```python
from build123d import *

# Parameters (mm, degrees)
SCHIZZO1_R                   = 10
ESTRUSIONE_ESTRUSIONE1_DEPTH = 20
SCHIZZO2_R                   = 3
ESTRUSIONE_ESTRUSIONE2_DEPTH = 13.2
SMUSSO1_SIZE                 = 0.5
FORO_FILETTATO_M10_3_D       = 8.5


with BuildPart() as part:
    # Schizzo1 → Estrusione-Estrusione1 (new body)
    with BuildSketch(Plane.XY):
        Circle(SCHIZZO1_R)
    extrude(amount=ESTRUSIONE_ESTRUSIONE1_DEPTH)

    # Schizzo2 → Estrusione-Estrusione2 (add, symmetric)
    with BuildSketch(Plane.XY.offset(10)):
        Circle(SCHIZZO2_R)
    extrude(amount=ESTRUSIONE_ESTRUSIONE2_DEPTH, both=True)

    # Smusso1
    smusso1_edges = [part.edges().sort_by_distance(p)[0] for p in [
        (-3, 0, -3.2),
        (-3, 0, 23.2),
    ]]
    chamfer(smusso1_edges, length=SMUSSO1_SIZE)

    # Foro filettato M10-3 (through all)
    with Locations(Plane(origin=(0, 10, 10), x_dir=(1, 0, 0), z_dir=(0, 1, 0))):
        with Locations((0, 0)):
            Hole(FORO_FILETTATO_M10_3_D / 2)


solid = part.part
```
Could you check a few things on this model? Use its own coordinates, in mm. A direction names the side the tool comes from. Round coordinates to 2 decimals unless told otherwise and drop trailing zeros. Loops run counter-clockwise (first coordinate to the right, second up) from the corner with the lowest first, then second, coordinate; pieces in that order, holes last. Notation, with made-up numbers: (45.5, -37) - (91.5, -37) arc R6 cw to (91.5, -31) - close; hole circle Ø5 at (32.5, -32). An arc over 180 degrees is marked (long way). Answer in a Markdown table with one row per item. Add a question column.
(1) If we section it at D-D (y = -6): Please give me the cut outline in (x, z), plus the area to 3 significant figures.
(2) I'm going to push flat-ended pins straight in: pin 1 (8 mm diameter, centred on y = -1, z = 15.5, fed in from -X); pin 2 (1 mm diameter, centred on x = 6, y = 3.5, fed in from -Z); pin 3 (1.5 mm diameter, centred on x = 4.5, z = 16, fed in from -Y); pin 4 (3 mm diameter, centred on x = 8, z = 15.5, fed in from -Y). Where does each tip first touch, or does it pass through?
(3) If we section it at B-B (x = 0): Please give me the cut outline in (y, z).
(4) If we mould it in two halves opening along Z, with no side actions, what happens to faces 1 (the face through (-3, 0, 21)), 2 (the face through (2.1, 2.4, 20)), 3 (the face through (0.92, -0.14, 14.15))? For each: pulls with the +Z half, pulls with the -Z half, needs draft (parallel to the pull), parting line crosses it, or undercut.
(5) For faces 4 (the face through (2.1, 2.4, 0)), 5 (the face through (0, 0, -3.2)), which set-ups out of +Z, -Z, +X, -X, +Y, -Y let a thin tool reach every point of the face, with its end or its side?
(6) If we section it at A-A (y = 0): Please give me the cut outline in (x, z), plus the area to 3 significant figures.
(7) I need wall thicknesses on line 1 along Z through (x, y) = (0, -5.5); line 2 along Z through (x, y) = (4.5, 8.25); line 3 along Y through (x, z) = (0.25, 18.25). Which ranges of each line are inside material? Lowest first, please.
(8) If we section it at C-C (z = 10): Please give me the cut outline in (x, y).
Model answer:
| question | item | result |
|---|---|---|
| 1 | outline | (-8, 0) - (8, 0) - (8, 20) - (-8, 20) - close; hole circle Ø8.5 at (0, 10) |
| 1 | area | 263 mm² |
| 2 | pin 1 | stops at x = -10 |
| 2 | pin 2 | stops at z = 0 |
| 2 | pin 3 | stops at y = -9.27 |
| 2 | pin 4 | stops at y = -7.6 |
| 3 | outline | (-10, 0) - (-3, 0) - (-3, -2.7) - (-2.5, -3.2) - (2.5, -3.2) - (3, -2.7) - (3, 0) - (10, 0) - (10, 5.75) - (-10, 5.75) - close; (-10, 14.25) - (10, 14.25) - (10, 20) - (3, 20) - (3, 22.7) - (2.5, 23.2) - (-2.5, 23.2) - (-3, 22.7) - (-3, 20) - (-10, 20) - close |
| 4 | face 1 | needs draft |
| 4 | face 2 | pulls with the +Z half |
| 4 | face 3 | undercut |
| 5 | face 4 | -Z |
| 5 | face 5 | -Z, +X, -X, +Y, -Y |
| 6 | outline | (-10, 0) - (-3, 0) - (-3, -2.7) - (-2.5, -3.2) - (2.5, -3.2) - (3, -2.7) - (3, 0) - (10, 0) - (10, 20) - (3, 20) - (3, 22.7) - (2.5, 23.2) - (-2.5, 23.2) - (-3, 22.7) - (-3, 20) - (-10, 20) - close; hole circle Ø8.5 at (0, 10) |
| 6 | area | 381 mm² |
| 7 | line 1 | z = 0 to 5.75, 14.25 to 20 |
| 7 | line 2 | z = 0 to 20 |
| 7 | line 3 | y = -10 to 10 |
| 8 | outline | (-4.25, -9.05) - (-4.25, 9.05) arc R10 ccw to start; (4.25, -9.05) arc R10 ccw to (4.25, 9.05) - close |
